Geometry: final body of the model. Coordinates: model frame, mm. A direction names the side the tool comes from. Round coordinates to 2 decimals unless told otherwise and drop trailing zeros. Order: outer loops, then holes, each group sorted by start corner. A loop starts at its lowest first (then second) coordinate and runs counter-clockwise, first axis right, second up. Notation, with made-up numbers: (-14, 22) - (-4, 22) arc R11 ccw to (-4, 37) - close; hole circle Ø2 at (0, 7.5). An arc over 180 degrees is marked (long way). Put each result on its own line as item: value. Start each with the question number.
(1) Section D-D (y = 0). Output: boundary loops of the cut face in (x, z), and give its area (3 significant figures).
(2) Access query for faces 4 (the face through (11, 0, 4)), 5 (the face through (7, 4, 10)), 6 (the face through (2, 0, 4)). Directions: +Z, -Z, +X, -X, +Y, -Y. A direction counts if a zero-diameter tool reaches every point of the face in a straight line with its end or side. Return the directions, or none.
(3) Material intervals for L1, parallel to Y at x = 7.75, z = 15; L2, parallel to Z at x = 10.75, y = -1; L3, parallel to Z at x = 9.25, y = -1, sorted ascending. Write a range as [from, to].
(4) Section C-C (x = 2.75). Output: boundary loops of the cut face in (y, z), and give its area (3 significant figures).
(5) Section A-A (z = 9). Output: boundary loops of the cut face in (x, y).
(6) Pull-direction query (Y, two-part tool) for faces 1 (the face through (7, -4, 10)), 2 (the face through (7.46, 0.05, 13.75)), 3 (the face through (6, 0, -2)); classes: released by +Y, released by -Y, zero draft, split by the parting line, or undercut.
(7) Section B-B (y = 2). Output: boundary loops of the cut face in (x, z).
(8) Pin query (flat end, axial travel): P1, Ø6, axis at x = 5.5, z = 6, coming from the +Y side; P2, Ø2.5, axis at y = 0.5, z = 12, coming from the +X side; P3, Ø0.5, axis at x = 11, y = 0.5, coming from the +Z side. Return the tip coordinate at first contact, or that it passes through.
from build123d import *

# Parameters (mm, degrees)
SKETCH1_R               = 1
SKETCH1_W               = 4
SKETCH1_H               = 8
BOSS_EXTRUDE1_DEPTH     = 12
SKETCH2_W               = 12
SKETCH2_H               = 8
BOSS_EXTRUDE2_DEPTH     = 2
SKETCH3_W               = 5
SKETCH3_H               = 8
BOSS_EXTRUDE3_DEPTH     = 15
SKETCH4_R               = 1.25
CUT_EXTRUDE1_DEPTH      = 6
CUT_EXTRUDE1_DEPTH_BACK = 8
FILLET1_R               = 0.2


with BuildPart() as part:
    # Sketch1 → Boss-Extrude1 (new body)
    with BuildSketch(Plane(origin=(0, 0, 0), x_dir=(0, 0, -1), z_dir=(1, 0, 0))):
        with Locations((0, -4)):
            Circle(SKETCH1_R)
        with Locations((0, 4)):
            Circle(SKETCH1_R)
        Rectangle(SKETCH1_W, SKETCH1_H)
        with BuildLine():
            ThreePointArc((-1, -4), (0, -5), (1, -4))
            Line((1, -4), (-1, -4))
        make_face()
        with BuildLine():
            Line((-1, -4), (1, -4))
            ThreePointArc((1, -4), (0, -3), (-1, -4))
        make_face()
    extrude(amount=BOSS_EXTRUDE1_DEPTH)

    # Sketch2 → Boss-Extrude2 (add)
    with BuildSketch(Plane.XY.offset(2)):
        with Locations((6, 0)):
            Rectangle(SKETCH2_W, SKETCH2_H)
    extrude(amount=BOSS_EXTRUDE2_DEPTH)

    # Sketch3 → Boss-Extrude3 (add)
    with BuildSketch(Plane.XY.offset(4)):
        with Locations((7.5, 0)):
            Rectangle(SKETCH3_W, SKETCH3_H)
    extrude(amount=BOSS_EXTRUDE3_DEPTH)

    # Sketch4 → Cut-Extrude1 (cut, two sides)
    with BuildSketch(Plane.ZY.offset(-5)) as cut_extrude1_sk:
        with Locations((15, 0)):
            Circle(SKETCH4_R)
        with Locations((9, 0)):
            Circle(SKETCH4_R)
    extrude(amount=CUT_EXTRUDE1_DEPTH, mode=Mode.SUBTRACT)
    extrude(cut_extrude1_sk.sketch, amount=-CUT_EXTRUDE1_DEPTH_BACK, mode=Mode.SUBTRACT)

    # Fillet1
    fillet1_edges = [part.edges().sort_by_distance(p)[0] for p in [
        (12, -5, 0),
        (0, -5, 0),
        (12, 5, 0),
        (0, 5, 0),
        (2.5, -4, 4),
        (5, -4, 11.5),
        (10, -4, 11.5),
        (11, -4, 4),
        (12, -4, 2.5),
        (6, -4, 1),
        (0, -4, 2.5),
        (10, 0, 19),
        (7.5, -4, 19),
        (5, 0, 19),
        (6, 4, 1),
        (12, 4, 2.5),
        (11, 4, 4),
        (10, 4, 11.5),
        (7.5, 4, 19),
        (5, 4, 11.5),
        (2.5, 4, 4),
        (0, 4, 2.5),
        (12, 0, 4),
        (10, 0, 4),
    ]]
    fillet(fillet1_edges, radius=FILLET1_R)


solid = part.part
Checks:
1. outline: (0, -2) - (12, -2) - (12, 3.8) arc R0.2 ccw to (11.8, 4) - (10.2, 4) arc R0.2 cw to (10, 4.2) - (10, 7.75) - (5, 7.75) - (5, 4) - (0, 4) - close; (5, 10.25) - (10, 10.25) - (10, 13.75) - (5, 13.75) - close; (5, 16.25) - (10, 16.25) - (10, 18.8) arc R0.2 ccw to (9.8, 19) - (5.2, 19) arc R0.2 ccw to (5, 18.8) - close
1. area: 122 mm²
2. face 4: +Z, +X, +Y, -Y
2. face 5: +Z, +X, -X, +Y
2. face 6: +Z, -X, +Y, -Y
3. L1: y = [-4, -1.25], [1.25, 4]
3. L2: z = [-2, 4]
3. L3: z = [-2, 8.25], [9.75, 14.25], [15.75, 19]
4. outline: (-4.17, 0.99) arc R1 ccw to (-4, -1) - (-4, -2) - (4, -2) - (4, -1) arc R1 ccw to (4.17, 0.99) arc R0.2 cw to (4, 1.18) - (4, 3.8) arc R0.2 ccw to (3.8, 4) - (-3.8, 4) arc R0.2 ccw to (-4, 3.8) - (-4, 1.18) arc R0.2 cw to start
4. area: 51.1 mm²
5. outline: (5, -3.8) arc R0.2 ccw to (5.2, -4) - (9.8, -4) arc R0.2 ccw to (10, -3.8) - (10, -1.25) - (5, -1.25) - close; (5, 1.25) - (10, 1.25) - (10, 3.8) arc R0.2 ccw to (9.8, 4) - (5.2, 4) arc R0.2 ccw to (5, 3.8) - close
6. face 1: released by -Y
6. face 2: undercut
6. face 3: zero draft
7. outline: (0, -2) - (12, -2) - (12, 3.8) arc R0.2 ccw to (11.8, 4) - (10.2, 4) arc R0.2 cw to (10, 4.2) - (10, 18.8) arc R0.2 ccw to (9.8, 19) - (5.2, 19) arc R0.2 ccw to (5, 18.8) - (5, 4) - (0, 4) - close
8. P1: stops at y = 4
8. P2: stops at x = 10
8. P3: stops at z = 4
